Work out the finished part from the listing and answer in its coordinate system (mm). A direction names the side the tool comes from. Give positions to 0.01 mm unless a question says otherwise; leave off trailing zeros. Order: outer loops, then holes, each group sorted by start corner. A loop starts at its lowest first (then second) coordinate and runs counter-clockwise, first axis right, second up. Notation, with made-up numbers: (-29, -36.75) - (-1, -36.75) arc R16 cw to (-1, -17.75) - close; hole circle Ø7 at (85, 46.25). An arc over 180 degrees is marked (long way). Return JSON: item names as keys, results as strings. Group by question number.
from build123d import *

# Parameters (mm, degrees)
SKETCH1_W           = 5
SKETCH1_H           = 10
BOSS_EXTRUDE1_DEPTH = 5
CUT_EXTRUDE1_DEPTH  = 10
CUT_EXTRUDE2_DEPTH  = 10


with BuildPart() as part:
    # Sketch1 → Boss-Extrude1 (new body)
    with BuildSketch(Plane(origin=(0, 0, 0), x_dir=(1, 0, 0), z_dir=(0, 1, 0))):
        with BuildLine():
            Line((0, 70), (0, -70))
            ThreePointArc((0, -70), (-70, 0), (0, 70))
        make_face()
        with Locations((-42.5, 0)):
            Rectangle(SKETCH1_W, SKETCH1_H, mode=Mode.SUBTRACT)
    extrude(amount=BOSS_EXTRUDE1_DEPTH)

    # Sketch2 → Cut-Extrude1 (cut)
    with BuildSketch(Plane(origin=(0, 5, 0), x_dir=(1, 0, 0), z_dir=(0, 1, 0))):
        Polygon((-7.6, -10), (-2.6, -10), (-2.6, 0), (-2.6, 10), (-7.6, 10), align=None)
    extrude(amount=-CUT_EXTRUDE1_DEPTH, mode=Mode.SUBTRACT)

    # Sketch3 → Cut-Extrude2 (cut)
    with BuildSketch(Plane(origin=(0, 5, 0), x_dir=(1, 0, 0), z_dir=(0, 1, 0))):
        Polygon((-28.6, 0), (-28.6, -10), (-33.6, -10), (-33.6, 10), (-28.6, 10), align=None)
    extrude(amount=-CUT_EXTRUDE2_DEPTH, mode=Mode.SUBTRACT)


solid = part.part
1. Each of these flat-tipped pins is pushed along its axis until it touches: pin 1 (1 mm diameter, centred on x = -8.5, y = 3, fed in from -Z); pin 2 (1.5 mm diameter, centred on y = 1.5, z = -1.5, fed in from -X); pin 3 (2.5 mm diameter, centred on x = -42.5, y = 3.5, fed in from -Z). Where does it stop, or does it pass through?
2. The part is cut by section D-D (z = -31.5). Give the vertices of the cut face in (x, y).
3. Consider probe 1 along X at (y, z) = (0.65, 0.5); probe 2 along X at (y, z) = (2.7, -3.5); probe 3 along Z at (x, y) = (-3, 4). Determine where each line is inside the solid, lowest interval first. Write a range as from..to.
4. A tool of negligible diameter and unlimited length cuts with its end or side. For faces 4 (the flat face through (-5, 3, -10)), 5 (the flat face through (0, 2, -1)), from which of +Z, -Z, +X, -X, +Y, -Y can it reach the whole face along a straight path? Write none if from no direction.
5. The part is cut by section A-A (z = 0). Give the vertices of the cut face in (x, y), and give its area (3 significant figures).
6. The part is cut by section C-C (x = -50.5). Give the vertices of the cut face in (y, z).
7. Determine the mould class of faces 1 (the cylindrical face through (-69.983, 2.465, 1.539)), 2 (the flat face through (-33.6, 3, 0)), 3 (the flat face through (-27, 0, -1)) for opening direction Z: released by +Z, released by -Z, zero draft, split by the parting line, or undercut.
8. The part is cut by section B-B (y = 3.2). Give the vertices of the cut face in (x, z).
Answers:
{
 "1": {"pin 1": "stops at z = -69.54", "pin 2": "stops at x = -70", "pin 3": "stops at z = -56.55"},
 "2": {"outline": "(-62.51, 0) - (0, 0) - (0, 5) - (-62.51, 5) - close"},
 "3": {"probe 1": "x = -70..-45, -40..-33.6, -28.6..-7.6, -2.6..0", "probe 2": "x = -69.91..-45, -40..-33.6, -28.6..-7.6, -2.6..0", "probe 3": "z = -69.94..-10, 10..69.94"},
 "4": {"face 4": "+Y, -Y", "face 5": "+Z, -Z, +X, +Y, -Y"},
 "5": {"outline": "(-70, 0) - (-45, 0) - (-45, 5) - (-70, 5) - close; (-40, 0) - (-33.6, 0) - (-33.6, 5) - (-40, 5) - close; (-28.6, 0) - (-7.6, 0) - (-7.6, 5) - (-28.6, 5) - close; (-2.6, 0) - (0, 0) - (0, 5) - (-2.6, 5) - close", "area": "275 mm^2"},
 "6": {"outline": "(0, -48.47) - (5, -48.47) - (5, 48.47) - (0, 48.47) - close"},
 "7": {"face 1": "split by the parting line", "face 2": "undercut", "face 3": "zero draft"},
 "8": {"outline": "(0, -70) - (0, 70) arc R70 ccw to start; hole (-45, -5) - (-40, -5) - (-40, 5) - (-45, 5) - close; hole (-33.6, -10) - (-28.6, -10) - (-28.6, 10) - (-33.6, 10) - close; hole (-7.6, -10) - (-2.6, -10) - (-2.6, 10) - (-7.6, 10) - close"}
}
